```python
from build123d import *

# Parameters (mm, degrees)
SKETCH1_W           = 127
SKETCH1_H           = 355.6
BOSS_EXTRUDE1_DEPTH = 4.445
SKETCH2_R           = 2.54
SKETCH2_R_2         = 14.2875
CUT_EXTRUDE1_DEPTH  = 190.008259343


with BuildPart() as part:
    # Sketch1 → Boss-Extrude1 (new, symmetric)
    with BuildSketch(Plane.XY):
        Rectangle(SKETCH1_W, SKETCH1_H)
    extrude(amount=BOSS_EXTRUDE1_DEPTH, both=True)

    # Sketch2 → Cut-Extrude1 (cut, through all)
    with BuildSketch(Plane.XY.offset(4.445)):
        with Locations((-31.75, -19.05)):
            Circle(SKETCH2_R)
        with Locations((-31.75, 19.05)):
            Circle(SKETCH2_R)
        with Locations((0, 10.125)):
            Circle(SKETCH2_R_2)
        with Locations((31.75, 19.05)):
            Circle(SKETCH2_R)
        with Locations((31.75, -19.05)):
            Circle(SKETCH2_R)
    extrude(amount=-CUT_EXTRUDE1_DEPTH, mode=Mode.SUBTRACT)


solid = part.part
```
For this review, take the finished solid that the model builds, in its own axes (mm). Coordinates: 2 decimals unless noted, no trailing zeros. Loops run counter-clockwise (first coordinate to the right, second up) from the corner with the lowest first, then second, coordinate; pieces in that order, holes last. Notation, with made-up numbers: (80, 84.5) -> (128, 84.5) arc R8 ccw to (128, 99.5) -> close; hole circle Ø7 at (-35, 72). An arc over 180 degrees is marked (long way). Return JSON: item names as keys, results as strings. Group by question number.
(1) Mouldability with a two-part tool opening along X and no side actions: class faces 1 (the flat face through (-63.5, -2, 0)), 2 (the flat face through (63.5, -2, 0)), 3 (the flat face through (13, 2, 4.445)), 4 (the cylindrical face through (-3.097, -3.823, 0.062)) as pulls with the +X half, pulls with the -X half, needs draft (parallel to the pull), parting line crosses it, or undercut.
(2) Consider section A-A, the plane x = 0. Give the boundary of the cut face in (y, z) (1 decimal).
(3) To check wall thickness, follow L1, parallel to Y at x = -31.75, z = 2.75; L2, parallel to Y at x = 0, z = 2.75; L3, parallel to Y at x = 1, z = -2. State the ranges of each line that lie inside material, in increasing order.
(4) Consider section B-B, the plane z = 0.75. Count the separate pieces of the cut face and the enclosed holes in it, plus the area to 3 significant figures.
Results below:
{
 "1": {"face 1": "pulls with the -X half", "face 2": "pulls with the +X half", "face 3": "needs draft", "face 4": "undercut"},
 "2": {"outline": "(-177.8, -4.4) -> (-4.2, -4.4) -> (-4.2, 4.4) -> (-177.8, 4.4) -> close; (24.4, -4.4) -> (177.8, -4.4) -> (177.8, 4.4) -> (24.4, 4.4) -> close"},
 "3": {"L1": "y = -177.8 to -21.59, -16.51 to 16.51, 21.59 to 177.8", "L2": "y = -177.8 to -4.16, 24.41 to 177.8", "L3": "y = -177.8 to -4.13, 24.38 to 177.8"},
 "4": {"separate pieces": "1", "enclosed holes": "5", "area": "44,400 mm2"}
}
